For this review, use the dimensioned drawing (mm, ordinates from the lowest corner) and the shaded views. Coordinates: 2 decimals unless noted, no trailing zeros. Order: outer loops, then holes, each group sorted by start corner. A loop starts at its lowest first (then second) coordinate and runs counter-clockwise, first axis right, second up. Notation, with made-up numbers: (-6.75, 42.5) -> (35.25, 42.5) arc R36 ccw to (35.25, 76.5) -> close; hole circle Ø2 at (59, -28.5). An arc over 180 degrees is marked (long way). Use one line per item in the form item = value. Start each with the question number.
(1) Wall thickness on line 1 along Z through (x, y) = (0.3, 3.75); line 2 along Z through (x, y) = (0.45, 9.75); line 3 along Y through (x, z) = (0.45, 1.5): over which ranges is each line inside the solid? List them lowest first.
(2) Take a section at D-D (z = 18.25). State the section outline as (x, y) points, then the cut area to 3 significant figures.
(3) Take a section at C-C (x = 0.85). State how many separate pieces and enclosed holes the cut face has, then the cut area to 3 significant figures.
(4) Take a section at A-A (y = 7.75). State the section outline as (x, z) points.
(5) Insertion check: pin 1 Ø1.2 at (y, z) = (5.75, 1.75) entering from -X; pin 2 Ø2.5 at (y, z) = (1.75, 5.75) entering from +X. Each pin has a flat end and moves straight along its axis. Give the tip position at first contact, or say it passes through.
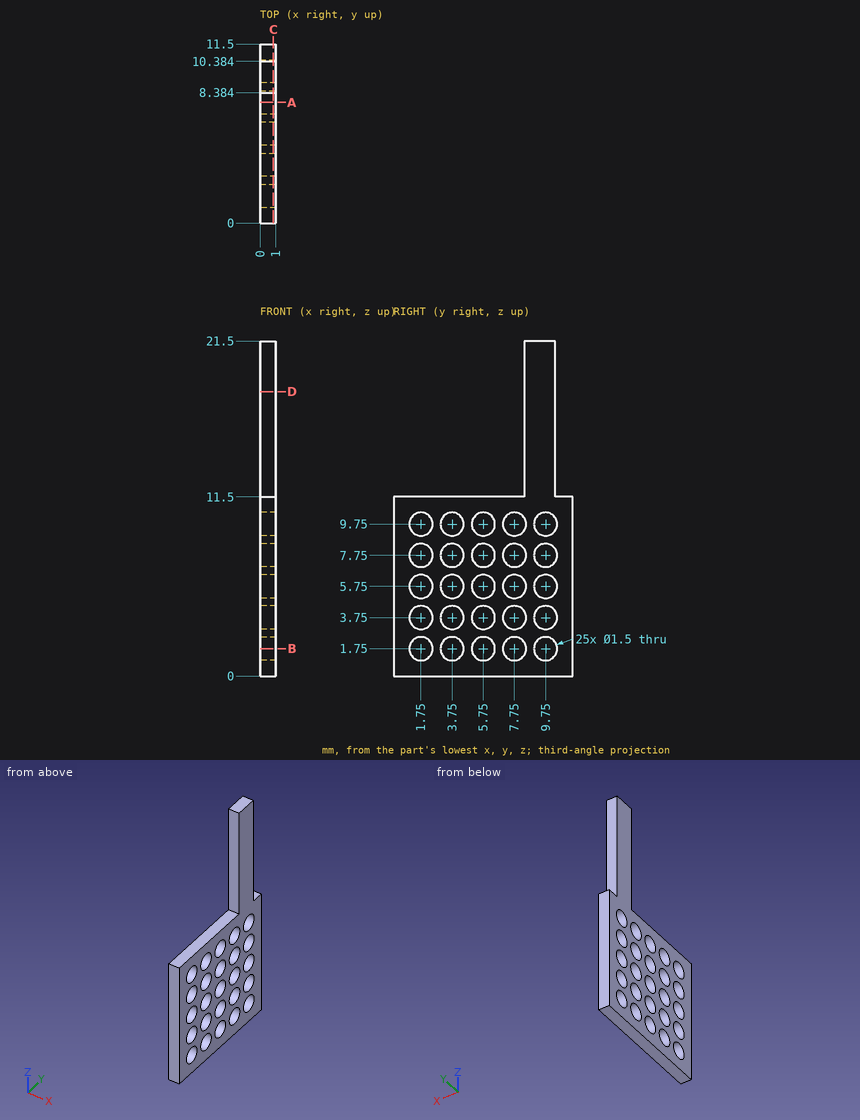
Findings:
q1.line_1 = 0 to 1, 2.5 to 3, 4.5 to 5, 6.5 to 7, 8.5 to 9, 10.5 to 11.5
q1.line_2 = 0 to 1, 2.5 to 3, 4.5 to 5, 6.5 to 7, 8.5 to 9, 10.5 to 21.5
q1.line_3 = 0 to 1.04, 2.46 to 3.04, 4.46 to 5.04, 6.46 to 7.04, 8.46 to 9.04, 10.46 to 11.5
q2.outline = (0, 8.38) -> (1, 8.38) -> (1, 10.38) -> (0, 10.38) -> close
q2.area = 2.00 mm²
q3.separate_pieces = 1
q3.enclosed_holes = 25
q3.area = 108 mm²
q4.outline = (0, 0) -> (1, 0) -> (1, 1) -> (0, 1) -> close; (0, 2.5) -> (1, 2.5) -> (1, 3) -> (0, 3) -> close; (0, 4.5) -> (1, 4.5) -> (1, 5) -> (0, 5) -> close; (0, 6.5) -> (1, 6.5) -> (1, 7) -> (0, 7) -> close; (0, 8.5) -> (1, 8.5) -> (1, 9) -> (0, 9) -> close; (0, 10.5) -> (1, 10.5) -> (1, 11.5) -> (0, 11.5) -> close
q5.pin_1 = through
q5.pin_2 = 1
